Geometry: final body of the model. Coordinates: model frame, mm. Face numbers are marked on the shaded views. A direction names the side the tool comes from. Give positions to 0.01 mm unless a question says otherwise; leave off trailing zeros. Loops run counter-clockwise (first coordinate to the right, second up) from the corner with the lowest first, then second, coordinate; pieces in that order, holes last. Notation, with made-up numbers: (2.25, 64) -> (18.25, 64) arc R16 cw to (18.25, 89) -> close; hole circle Ø5 at (64.25, 88). An arc over 180 degrees is marked (long way). One line per item, written item: value. Start each with the question number.
from build123d import *

# Parameters (mm, degrees)
SKETCH2_R           = 5
BOSS_EXTRUDE1_DEPTH = 22
CUT_EXTRUDE1_START  = -6
SKETCH3_R           = 5
SKETCH3_R_2         = 2.45
CUT_EXTRUDE1_DEPTH  = 6
SKETCH4_R           = 5
SKETCH4_R_2         = 2.45
CUT_EXTRUDE2_DEPTH  = 6


with BuildPart() as part:
    # Sketch2 → Boss-Extrude1 (new body)
    with BuildSketch(Plane(origin=(0, 0, 0), x_dir=(1, 0, 0), z_dir=(0, 1, 0))):
        with Locations(Location((0, 0, 0), (0, 0, 270))):
            Circle(SKETCH2_R)
    extrude(amount=BOSS_EXTRUDE1_DEPTH)

    # Sketch3 → Cut-Extrude1 (cut)
    with BuildSketch(Plane(origin=(0, 22, 0), x_dir=(1, 0, 0), z_dir=(0, 1, 0)).offset(CUT_EXTRUDE1_START)):
        with Locations(Location((0, 0, 0), (0, 0, 270))):
            Circle(SKETCH3_R)
        with Locations(Location((0, 0, 0), (0, 0, 270))):
            Circle(SKETCH3_R_2, mode=Mode.SUBTRACT)
    extrude(amount=CUT_EXTRUDE1_DEPTH, mode=Mode.SUBTRACT)

    # Sketch4 → Cut-Extrude2 (cut)
    with BuildSketch(Plane.XZ):
        with Locations(Location((0, 0, 0), (0, 0, 270))):
            Circle(SKETCH4_R)
        with Locations(Location((0, 0, 0), (0, 0, 90))):
            Circle(SKETCH4_R_2, mode=Mode.SUBTRACT)
    extrude(amount=-CUT_EXTRUDE2_DEPTH, mode=Mode.SUBTRACT)


solid = part.part
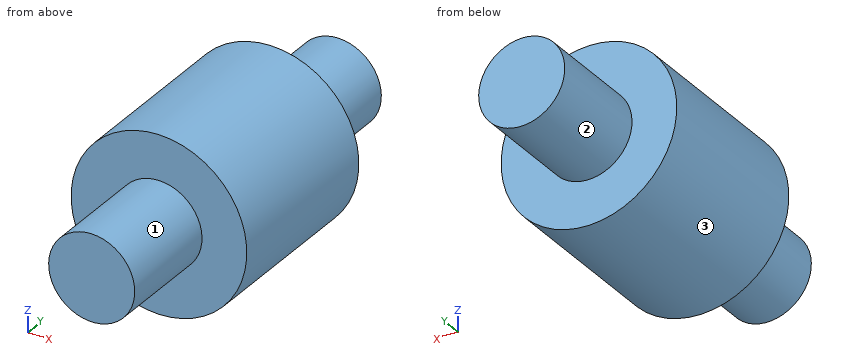
Item 1: Section C-C, the plane y = 7.75. Output: boundary loops of the cut face in (x, z), then the cut area to 3 significant figures.
Item 2: Section B-B, the plane z = 0. Output: boundary loops of the cut face in (x, y).
Item 3: Section A-A, the plane x = 0. Output: boundary loops of the cut face in (y, z), then the cut area to 3 significant figures.
Item 4: Section D-D, the plane y = 1.5. Output: boundary loops of the cut face in (x, z).
Item 5: Ray query, line 1 along Y through (x, z) = (-3.25, -0.5); line 2 along X through (y, z) = (7, 3); line 3 along Z through (x, y) = (-0.5, 12). Return the intervals inside material, ascending. Write a range as [from, to].
Item 6: Access query for the marked faces 1, 2 and 3. Directions: +Z, -Z, +X, -X, +Y, -Y. A direction counts if a zero-diameter tool reaches every point of the face in a straight line with its end or side. Return the directions, or none.
Item 7: Pin query (flat end, axial travel): pin 1 (1.5 mm diameter, centred on x = -1, z = -1, fed in from -Y); pin 2 (2 mm diameter, centred on x = -3, y = 8.5, fed in from +Z); pin 3 (6 mm diameter, centred on y = 5, z = 3.5, fed in from -X); pin 4 (1 mm diameter, centred on y = 17, z = -1.5, fed in from +X). Return the tip coordinate at first contact, or that it passes through.
Geometry check:
1. outline: circle Ø10 at (0, 0)
1. area: 78.5 mm2
2. outline: (-5, 6) -> (-2.45, 6) -> (-2.45, 0) -> (2.45, 0) -> (2.45, 6) -> (5, 6) -> (5, 16) -> (2.45, 16) -> (2.45, 22) -> (-2.45, 22) -> (-2.45, 16) -> (-5, 16) -> close
3. outline: (0, -2.45) -> (6, -2.45) -> (6, -5) -> (16, -5) -> (16, -2.45) -> (22, -2.45) -> (22, 2.45) -> (16, 2.45) -> (16, 5) -> (6, 5) -> (6, 2.45) -> (0, 2.45) -> close
3. area: 159 mm2
4. outline: circle Ø4.9 at (0, 0)
5. line 1: y = [6, 16]
5. line 2: x = [-4, 4]
5. line 3: z = [-4.97, 4.97]
6. face 1: -Y
6. face 2: +Y
6. face 3: +Y, -Y
7. pin 1: stops at y = 0
7. pin 2: stops at z = 4.58
7. pin 3: stops at x = -4.95
7. pin 4: stops at x = 2.24
